```python
from build123d import *

# Parameters (mm, degrees)
PAD_DEPTH    = 80
FILLET_R     = 10
SKETCH001_R  = 38
PAD001_DEPTH = 160


with BuildPart() as part:
    # Sketch → Pad (new body)
    with BuildSketch(Plane.XZ):
        Polygon((-62.473045, -51.467136), (67.526955, -51.467136), (67.526955, 28.532864), (27.526955, 28.532864), (13.0149, 43.531436), (-6.9851, 43.531436), (-22.473045, 28.532864), (-62.473045, 28.532864), align=None)
    extrude(amount=PAD_DEPTH)

    # Fillet
    fillet_edges = [part.edges().sort_by_distance(p)[0] for p in [
        (27.526955, -40, 28.532864),
        (-22.473045, -40, 28.532864),
        (-6.9851, -40, 43.531436),
        (13.0149, -40, 43.531436),
        (-62.473045, -40, 28.532864),
        (67.526955, -40, 28.532864),
        (67.526955, -40, -51.467136),
        (-62.473045, -40, -51.467136),
        (-62.473045, -80, -11.467136),
        (2.526955, -80, -51.467136),
        (67.526955, -80, -11.467136),
        (67.526955, 0, -11.467136),
        (2.526955, 0, -51.467136),
        (47.526955, 0, 28.532864),
        (20.270928, 0, 36.03215),
        (3.0149, 0, 43.531436),
        (-14.729072, 0, 36.03215),
        (-42.473045, 0, 28.532864),
        (-62.473045, 0, -11.467136),
        (-42.473045, -80, 28.532864),
        (-14.729072, -80, 36.03215),
        (3.0149, -80, 43.531436),
        (20.270928, -80, 36.03215),
        (47.526955, -80, 28.532864),
    ]]
    fillet(fillet_edges, radius=FILLET_R)

    # Sketch001 → Pad001 (join)
    with BuildSketch(Plane.XZ):
        with Locations((3.063112, -10.729656)):
            Circle(SKETCH001_R)
    extrude(amount=PAD001_DEPTH)


solid = part.part
```
Geometry: final body of the model. Coordinates: model frame, mm. A direction names the side the tool comes from. Coordinates: 2 decimals unless noted, no trailing zeros. Order: outer loops, then holes, each group sorted by start corner. A loop starts at its lowest first (then second) coordinate and runs counter-clockwise, first axis right, second up. Notation, with made-up numbers: (41, -18.5) -> (82, -18.5) arc R34 cw to (82, 17.5) -> close; hole circle Ø6 at (14.25, 35). An arc over 180 degrees is marked (long way). Answer in a Markdown table with one row per item.
Item 1: Access query for faces 1 (the cylindrical face through (3.3, -4.35, -49.72)), 2 (the cylindrical face through (-39.679, -76.993, 25.681)), 3 (the flat face through (3, -160, -10)), 4 (the cylindrical face through (-39.679, -3.007, 25.681)), 5 (the cylindrical face through (-27.092, -117.855, -33.852)). Directions: +Z, -Z, +X, -X, +Y, -Y. A direction counts if a zero-diameter tool reaches every point of the face in a straight line with its end or side. Return the directions, or none.
Return value:
| item | result |
|---|---|
| face 1 | -Z, +Y |
| face 2 | +Z, -X, -Y |
| face 3 | +Z, -Z, +X, -X, -Y |
| face 4 | +Z, -X, +Y |
| face 5 | -Y |
Item 2: Section D-D on z = 10. Output: boundary loops of the cut face in (x, y).
Return value:
| item | result |
|---|---|
| outline | (-62.47, -70) arc R10 ccw to (-52.47, -80) -> (-28.78, -80) -> (-28.78, -160) -> (34.91, -160) -> (34.91, -80) -> (57.53, -80) arc R10 ccw to (67.53, -70) -> (67.53, -10) arc R10 ccw to (57.53, 0) -> (-52.47, 0) arc R10 ccw to (-62.47, -10) -> close |
Item 3: Section B-B on y = -56.5. Output: boundary loops of the cut face in (x, z).
Return value:
| item | result |
|---|---|
| outline | (-62.47, -41.47) arc R10 ccw to (-52.47, -51.47) -> (57.53, -51.47) arc R10 ccw to (67.53, -41.47) -> (67.53, 18.53) arc R10 ccw to (57.53, 28.53) -> (31.77, 28.53) arc R10 cw to (24.58, 31.58) -> (15.96, 40.48) arc R10 ccw to (8.78, 43.53) -> (-2.94, 43.53) arc R10 ccw to (-9.89, 40.72) -> (-19.56, 31.35) arc R10 cw to (-26.52, 28.53) -> (-52.47, 28.53) arc R10 ccw to (-62.47, 18.53) -> close |
Item 4: Section C-C on z = -39. Output: boundary loops of the cut face in (x, y).
Return value:
| item | result |
|---|---|
| outline | (-62.47, -70) arc R10 ccw to (-52.47, -80) -> (-22.33, -80) -> (-22.33, -160) -> (28.46, -160) -> (28.46, -80) -> (57.53, -80) arc R10 ccw to (67.53, -70) -> (67.53, -10) arc R10 ccw to (57.53, 0) -> (-52.47, 0) arc R10 ccw to (-62.47, -10) -> close |
Item 5: Ray query, L1, parallel to Y at x = -33.5, z = 12; L2, parallel to Z at x = 33, y = -44.5; L3, parallel to Z at x = -12, y = -145. Return the intervals inside material, ascending.
Return value:
| item | result |
|---|---|
| L1 | y = -80 to 0 |
| L2 | z = -51.47 to 28.53 |
| L3 | z = -45.62 to 24.16 |
Item 6: Contact query for flat-ended pins moving along their axis: P1, Ø8, axis at y = -133.5, z = -2, coming from the -X side; P2, Ø4, axis at x = 9.5, y = -125, coming from the +Z side; P3, Ø13, axis at x = 43, y = -29.5, coming from the +Z side. Output: stop coordinate, or through.
Return value:
| item | result |
|---|---|
| P1 | stops at x = -34.64 |
| P2 | stops at z = 27.01 |
| P3 | stops at z = 28.53 |
Item 7: Section A-A on x = -44. Output: boundary loops of the cut face in (y, z), plus the area to 3 significant figures.
Return value:
| item | result |
|---|---|
| outline | (-80, -41.47) arc R10 ccw to (-70, -51.47) -> (-10, -51.47) arc R10 ccw to (0, -41.47) -> (0, 18.53) arc R10 ccw to (-10, 28.53) -> (-70, 28.53) arc R10 ccw to (-80, 18.53) -> close |
| area | 6,310 mm² |
